from build123d import *

# Parameters (mm, degrees)
SKETCH2_R           = 20
BOSS_EXTRUDE1_DEPTH = 5
SKETCH3_R           = 11.5
BOSS_EXTRUDE2_DEPTH = 65.062198088
FILLET3_R           = 10
FILLET5_R           = 5
SKETCH6_R           = 5.292916783
CUT_EXTRUDE1_DEPTH  = 85.504906147


with BuildPart() as part:
    # Sketch2 → Boss-Extrude1 (new body)
    with BuildSketch(Plane(origin=(0, 0, 0), x_dir=(0, 0, -1), z_dir=(1, 0, 0))):
        Circle(SKETCH2_R)
    extrude(amount=BOSS_EXTRUDE1_DEPTH)

    # Sketch3 → Boss-Extrude2 (add)
    with BuildSketch(Plane(origin=(5, 0, 0), x_dir=(0, 0, -1), z_dir=(1, 0, 0))):
        Circle(SKETCH3_R)
    extrude(amount=BOSS_EXTRUDE2_DEPTH)

    # Fillet3
    fillet3_edges = [part.edges().sort_by_distance(p)[0] for p in [
        (70.062198088, 0, 11.5),
    ]]
    fillet(fillet3_edges, radius=FILLET3_R)

    # Fillet5
    fillet5_edges = [part.edges().sort_by_distance(p)[0] for p in [
        (5, 0, 11.5),
    ]]
    fillet(fillet5_edges, radius=FILLET5_R)

    # Sketch6 → Cut-Extrude1 (cut, through all)
    with BuildSketch(Plane.XY.offset(22.806162663)):
        with Locations((51.062198088, 0)):
            Circle(SKETCH6_R)
    extrude(amount=-CUT_EXTRUDE1_DEPTH, mode=Mode.SUBTRACT)


solid = part.part
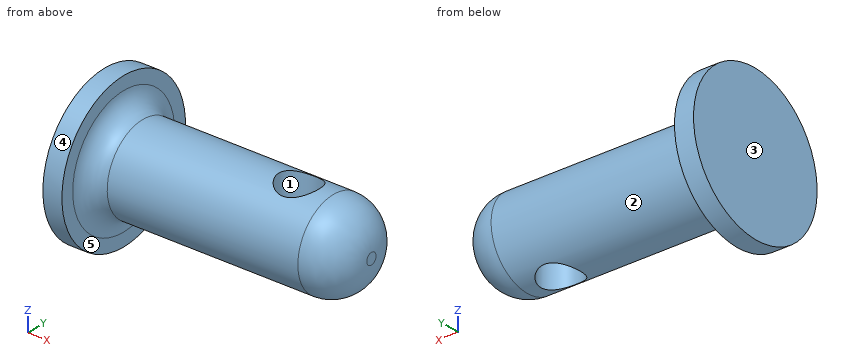
Model file for the job. Use its own axes, mm. Face numbers are marked on the shaded views. A direction names the side the tool comes from. Give positions to 0.01 mm unless a question says otherwise; leave off trailing zeros. Order: outer loops, then holes, each group sorted by start corner. A loop starts at its lowest first (then second) coordinate and runs counter-clockwise, first axis right, second up. Notation, with made-up numbers: (-16.75, 39.25) - (24.25, 39.25) arc R19 cw to (24.25, 46.25) - close; hole circle Ø6 at (-8.75, 18). An arc over 180 degrees is marked (long way). Return JSON: item names as keys, results as strings.
1) Cut at A-A, the plane x = 25.5. Give the cut face in (y, z).
Geometry says:
{"outline": "circle Ø23 at (0, 0)"}
2) 3-axis set-ups, long thin cutter, end or side, ignore diameter. For the marked faces 4 and 5: which of +Z, -Z, +X, -X, +Y, -Y reach the whole face in a straight line?
Geometry says:
{"face 4": "+X, -X", "face 5": "+X"}
3) Flat gauge pins, fed straight in: P1, Ø12, axis at x = 51.06, y = 0, coming from the -Z side; P2, Ø4, axis at x = 9.5, z = -5, coming from the -Y side; P3, Ø8, axis at x = 14, y = 0, coming from the +Z side; P4, Ø1.5, axis at x = 33.5, y = -12.5, coming from the -Z side. Where does each tip first touch, or does it go through?
Geometry says:
{"P1": "z = -11.5", "P2": "y = -11.34", "P3": "z = 11.5", "P4": "through"}
4) Pull direction Y, two halves, no side cores. Call the marked faces 1, 2 and 3: pulls with the +Y half, pulls with the -Y half, needs draft (parallel to the pull), parting line crosses it, or undercut.
Geometry says:
{"face 1": "undercut", "face 2": "parting line crosses it", "face 3": "needs draft"}
5) Probe line 1 (X direction, y = 0, z = -1.5); line 2 (Z direction, x = 35, y = 0.5); line 3 (X direction, y = -2.5, z = 6.5). List the from-to ranges inside material, lowest first. Write a range as from..to.
Geometry says:
{"line 1": "0..45.77, 56.36..70.06", "line 2": "-11.49..11.49", "line 3": "0..46.4, 55.73..68.44"}
